```python
from build123d import *

# Parameters (mm, degrees)
F0_R     = 2.25
F1_DEPTH = 15
F2_R     = 15.5
F3_DEPTH = 1


with BuildPart() as f1:
    # F0 (on Front) → F1 (new body)
    with BuildSketch(Plane.XZ):
        with BuildLine():
            add(Edge.make_bspline(
                [(50.3479777806, -2.8862454928), (53.268195878, -3.261348037), (58.6611963596, -3.9533176417), (62.2933460238, -6.1636902612), (63.9588082608, -7.1761531808)],
                knots=[0, 0, 0, 0, 0.5415192792, 1, 1, 1, 1], degree=3))
            Line((50.3479777806, -2.8862454928), (25.0282175839, -2.8862454928))
            Line((25.0282175839, -2.8862454928), (25.0282175839, -22.7884277701))
            Line((25.0282175839, -22.7884277701), (29.7951731688, -22.7884277701))
            ThreePointArc((29.7951731688, -22.7884277701), (28.4636985284, -31.7867677512), (30.8986199162, -40.5511333853))
            add(Edge.make_bspline(
                [(29.8397061446, -48.0479822571), (30.7470532857, -47.0116302158), (32.6276335059, -44.8769054108), (31.4765020534, -42.024639753), (30.8986199162, -40.5511333853)],
                knots=[0, 0, 0, 0, 0.485392469, 1, 1, 1, 1], degree=3))
            ThreePointArc((29.8397061446, -48.0479822571), (29.9610414714, -52.9277231917), (34.8411419508, -52.8218309708))
            add(Edge.make_bspline(
                [(34.8411419508, -52.8218309708), (34.9156373522, -52.7356864932), (34.9901022249, -52.6494127513), (35.065109933, -52.5643533984)],
                knots=[0, 0, 0, 0, 0.0825218812, 0.0825218812, 0.0825218812, 0.0825218812], degree=3))
            add(Edge.make_bspline(
                [(35.065109933, -52.5643533984), (35.4412326082, -52.1378272164), (36.3054316166, -51.2598405123), (37.5921223548, -51.3648089629), (38.303234242, -51.4084192455)],
                knots=[0.0825218812, 0.0825218812, 0.0825218812, 0.0825218812, 0.4963240293, 1, 1, 1, 1], degree=3))
            ThreePointArc((38.303234242, -51.4084192455), (44.0362215273, -53.6423292578), (50.1387902983, -54.4272824743))
            Line((50.1387902983, -54.4272824743), (50.4479777806, -54.4272824743))
            ThreePointArc((50.4479777806, -54.4272824743), (72.3721230889, -41.4992868245), (71.9812678774, -16.0503487087))
            add(Edge.make_bspline(
                [(72.8356159841, -9.4444898754), (71.9013864052, -10.6696925545), (70.5245996547, -12.8306913276), (71.3883715318, -15.0658070668), (71.9812678774, -16.0503487087)],
                knots=[0, 0, 0, 0, 0.524822635, 1, 1, 1, 1], degree=3))
            ThreePointArc((72.8356159841, -9.4444898754), (72.3990680605, -4.9396508075), (67.8742152822, -5.0389304732))
            add(Edge.make_bspline(
                [(67.8742152822, -5.0389304732), (66.812715433, -6.0682372602), (65.5657418957, -7.1263163681), (64.1965142668, -7.1894367778), (63.9588082608, -7.1761531808)],
                knots=[0, 0, 0, 0, 0.5190595992, 0.6268019641, 0.6268019641, 0.6268019641, 0.6268019641], degree=3))
        make_face()
        with Locations((32.3479777806, -50.4269927665)):
            Circle(F0_R, mode=Mode.SUBTRACT)
        with BuildLine():
            ThreePointArc((50.3479777806, -14.9272824743), (61.308132889, -19.4671273659), (65.8479777806, -30.4272824743))
            ThreePointArc((65.8479777806, -30.4272824743), (39.3878226722, -41.3874375827), (50.3479777806, -14.9272824743))
        make_face(mode=Mode.SUBTRACT)
        with Locations((70.1901335806, -7.4272824743)):
            Circle(F0_R, mode=Mode.SUBTRACT)
        with BuildLine():
            ThreePointArc((50.3479777806, -14.9272824743), (39.3878226722, -41.3874375827), (65.8479777806, -30.4272824743))
            ThreePointArc((65.8479777806, -30.4272824743), (61.308132889, -19.4671273659), (50.3479777806, -14.9272824743))
        make_face()
        with BuildLine():
            ThreePointArc((63.3479777806, -30.4272824743), (41.1555896252, -39.6196706298), (50.3479777806, -17.4272824743))
            ThreePointArc((50.3479777806, -17.4272824743), (59.5403659361, -21.2348943189), (63.3479777806, -30.4272824743))
        make_face(mode=Mode.SUBTRACT)
        with BuildLine():
            ThreePointArc((63.3479777806, -30.4272824743), (59.5403659361, -21.2348943189), (50.3479777806, -17.4272824743))
            ThreePointArc((50.3479777806, -17.4272824743), (41.1555896252, -39.6196706298), (63.3479777806, -30.4272824743))
        make_face()
        with BuildLine():
            add(Edge.make_bspline(
                [(34.8411419508, -52.8218309708), (34.9156373522, -52.7356864932), (34.9901022249, -52.6494127513), (35.065109933, -52.5643533984)],
                knots=[0, 0, 0, 0, 0.0825218812, 0.0825218812, 0.0825218812, 0.0825218812], degree=3))
            ThreePointArc((34.8411419508, -52.8218309708), (34.956304949, -52.6958574577), (35.065109933, -52.5643533984))
        make_face()
        with BuildLine():
            ThreePointArc((50.1387902983, -54.4272824743), (50.2933840395, -54.4277544812), (50.4479777806, -54.4272824743))
            Line((50.4479777806, -54.4272824743), (50.1387902983, -54.4272824743))
        make_face()
    extrude(amount=F1_DEPTH)

    # F2 (on face) → F3 (cut)
    with BuildSketch(Plane.XZ.offset(15)):
        with Locations((50.3479777806, -30.4272824743)):
            Circle(F2_R)
    extrude(amount=-F3_DEPTH, mode=Mode.SUBTRACT)


solid = f1.part
```
Verification items for the finished model (mm, model axes). A direction names the side the tool comes from. Give positions to 0.01 mm unless a question says otherwise; leave off trailing zeros. Loops run counter-clockwise (first coordinate to the right, second up) from the corner with the lowest first, then second, coordinate; pieces in that order, holes last. Notation, with made-up numbers: M 84.25,-32 L 99.25,-32 A32 cw 99.25,-4 Z; hole C 46.5,54.25 d6. An arc over 180 degrees is marked long. Return JSON: item names as keys, results as strings.
1) Gauge pin test, flat ends, axial feed: P1, Ø1, axis at y = -5, z = -49, coming from the +X side; P2, Ø1.5, axis at y = -8.5, z = -28, coming from the +X side; P3, Ø9.5, axis at x = 55, z = -34, coming from the -Y side; P4, Ø3.5, axis at x = 32.35, z = -50.43, coming from the -Y side. Record the tip position at first contact, or that the pin passes through.
Findings:
{"P1": "stops at x = 66.57", "P2": "stops at x = 75.61", "P3": "stops at y = -14", "P4": "passes through"}
2) Section check B-B, the plane x = 49. Enter the section's corners in (y, z), and give its area (3 significant figures).
Findings:
{"outline": "M -15,-54.39 L 0,-54.39 L 0,-2.89 L -15,-2.89 L -15,-14.99 L -14,-14.99 L -14,-45.87 L -15,-45.87 Z", "area": "742 mm2"}
3) Mould release check, pull along X, two halves, no side actions. Record for faces 3 (the flat face through (50, -14, -30)), 4 (the flat face through (27, -7, -22.788)), 5 (the cylindrical face through (72.451, -7.395, -4.986)), 6 (the flat face through (25.028, -7, -13)): released by +X, released by -X, zero draft, split by the parting line, or undercut.
Findings:
{"face 3": "undercut", "face 4": "zero draft", "face 5": "undercut", "face 6": "released by -X"}
4) Tool access check on faces 1 (the flat face through (39, -15, -17)), 2 (the cylindrical face through (38.924, -14.507, -19.952)). Record the directions out of +Z, -Z, +X, -X, +Y, -Y that give a thin tool (end or side, any length) a straight path to the whole face; none if there is none.
Findings:
{"face 1": "+Z, -Z, +X, -X, -Y", "face 2": "-Y"}
5) Section check C-C, the plane y = -3.5. Count the separate pieces of the cut face and the enclosed holes in it, and give its area (3 significant figures).
Findings:
{"separate pieces": "1", "enclosed holes": "2", "area": "2,160 mm2"}
6) Section check A-A, the plane z = -28.5. Enter the section's corners in (x, y).
Findings:
{"outline": "M 28.51,-15 L 34.97,-15 L 34.97,-14 L 65.73,-14 L 65.73,-15 L 75.6,-15 L 75.6,0 L 28.51,0 Z"}
7) Material ranges on L1, parallel to Z at x = 72, y = -2.75; L2, parallel to X at y = -8.5, z = -51; L3, parallel to X at y = -8.75, z = -50, recorded low to high. Write a range as [from, to].
Findings:
{"L1": "z = [-42.14, -16.08], [-10.62, -8.76], [-6.09, -4.64]", "L2": "x = [28.94, 30.17], [34.52, 63.01]", "L3": "x = [28.92, 30.14], [34.56, 64.6]"}
